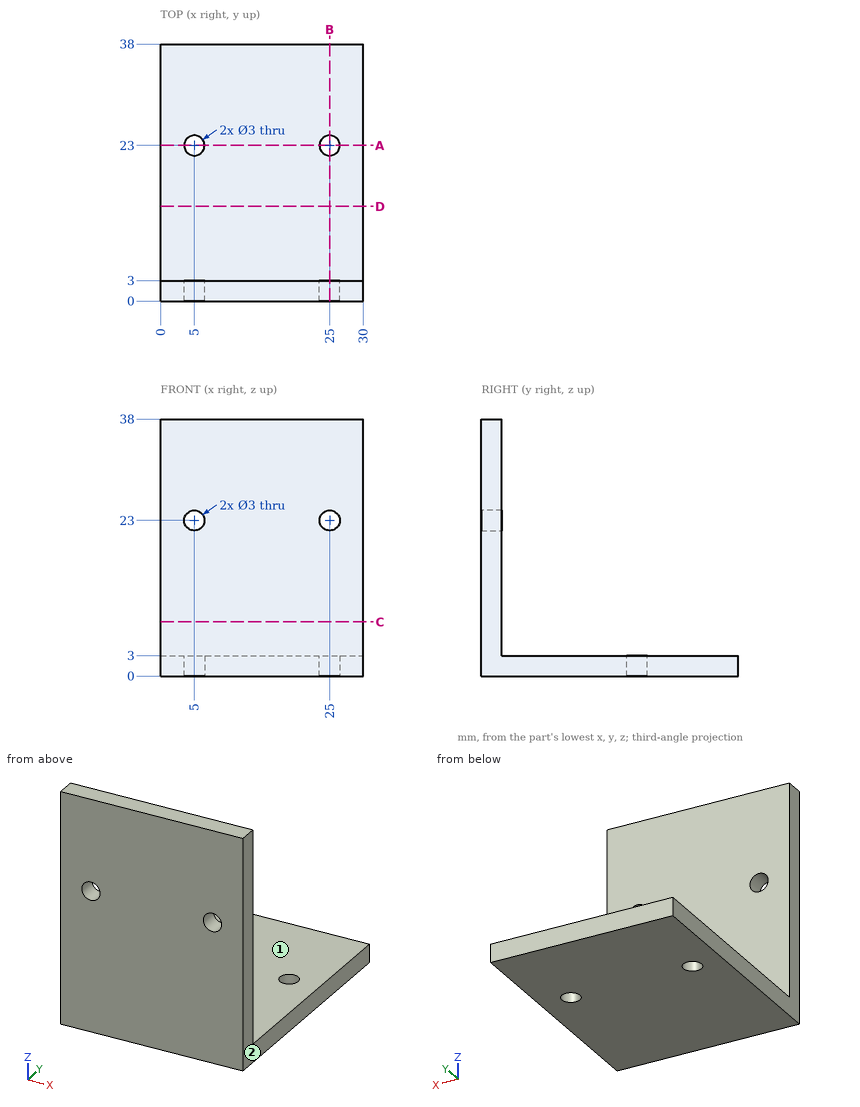
Design review of the part shown in the three views and the two pictorial views. Dimensions are in mm from the part's minimum x, y and z. A direction names the side the tool comes from. Round coordinates to 2 decimals unless told otherwise and drop trailing zeros. Loops run counter-clockwise (first coordinate to the right, second up) from the corner with the lowest first, then second, coordinate; pieces in that order, holes last. Notation, with made-up numbers: M 49.5,-19.75 L 56.5,-19.75 A10 ccw 56.5,-1.75 Z; hole C 5.5,9 d10. An arc over 180 degrees is marked long. Answer as a JSON object with one key per item and string values.
Item 1: Tool access review of the marked faces 1 and 2: name each direction out of +Z, -Z, +X, -X, +Y, -Y from which nothing blocks a thin tool from reaching the whole face with its end or side.
Check sheet entries:
{"face 1": "+Z, +X, -X, +Y", "face 2": "+Z, -Z, +X, +Y, -Y"}
Item 2: Clearance check with flat-ended pins moving along their axes: P1, Ø2.5, axis at x = 25, z = 23, coming from the +Y side; P2, Ø4, axis at x = 6.5, y = 24, coming from the +Z side; P3, Ø8, axis at x = 11.5, z = 15, coming from the +Y side. State where each tip first meets the part, or that it passes through.
Check sheet entries:
{"P1": "through", "P2": "z = 3", "P3": "y = 3"}
Item 3: We need section A-A, the plane y = 23. State the section outline as (x, z) points.
Check sheet entries:
{"outline": "M 0,0 L 3.5,0 L 3.5,3 L 0,3 Z; M 6.5,0 L 23.5,0 L 23.5,3 L 6.5,3 Z; M 26.5,0 L 30,0 L 30,3 L 26.5,3 Z"}
Item 4: For line 1 along X through (y, z) = (2, 23); line 2 along Y through (x, z) = (5, 2.45); line 3 along Y through (x, z) = (21, 7), list the stretches that pass through material, from the lowest coordinate up.
Check sheet entries:
{"line 1": "0 to 3.5, 6.5 to 23.5, 26.5 to 30", "line 2": "0 to 21.5, 24.5 to 38", "line 3": "0 to 3"}
Item 5: We need section B-B, the plane x = 25. State the section outline as (y, z) points, and give its area (3 significant figures).
Check sheet entries:
{"outline": "M 0,0 L 21.5,0 L 21.5,3 L 3,3 L 3,21.5 L 0,21.5 Z; M 0,24.5 L 3,24.5 L 3,38 L 0,38 Z; M 24.5,0 L 38,0 L 38,3 L 24.5,3 Z", "area": "201 mm2"}
Item 6: We need section C-C, the plane z = 8. State the section outline as (x, y) points.
Check sheet entries:
{"outline": "M 0,0 L 30,0 L 30,3 L 0,3 Z"}
